Part print with two shaded views. Sizes in mm from the minimum x, y, z corner. Give positions to 0.01 mm unless a question says otherwise; leave off trailing zeros. Order: outer loops, then holes, each group sorted by start corner. A loop starts at its lowest first (then second) coordinate and runs counter-clockwise, first axis right, second up. Notation, with made-up numbers: M 15,81.25 L 43,81.25 A32 ccw 43,116.25 Z; hole C 83.5,-22.5 d4. An arc over 180 degrees is marked long. Return JSON: item names as keys, results as strings. Group by question number.
1. Slice it at B-B on z = 120. List the corners of the cut face in (x, y) (3 decimals).
2. Pin check, flat tips, straight feed: pin 1 (1 mm diameter, centred on x = 158.5, y = 2, fed in from -Z) (3 decimals); pin 2 (1 mm diameter, centred on y = 2, z = 59, fed in from +X) (3 decimals); pin 3 (0.7 mm diameter, centred on x = 2, y = 1, fed in from -Z). Stop position of each tip, or through.
3. Wall check: probe 1 along Z at (x, y) = (83, 2.3) (3 decimals); probe 2 along X at (y, z) = (0.7, 117.5) (3 decimals). Give the ranges that are in metal, low to high. Write a range as [from, to].
4. Slice it at A-A on x = 119. List the corners of the cut face in (y, z) (3 decimals).
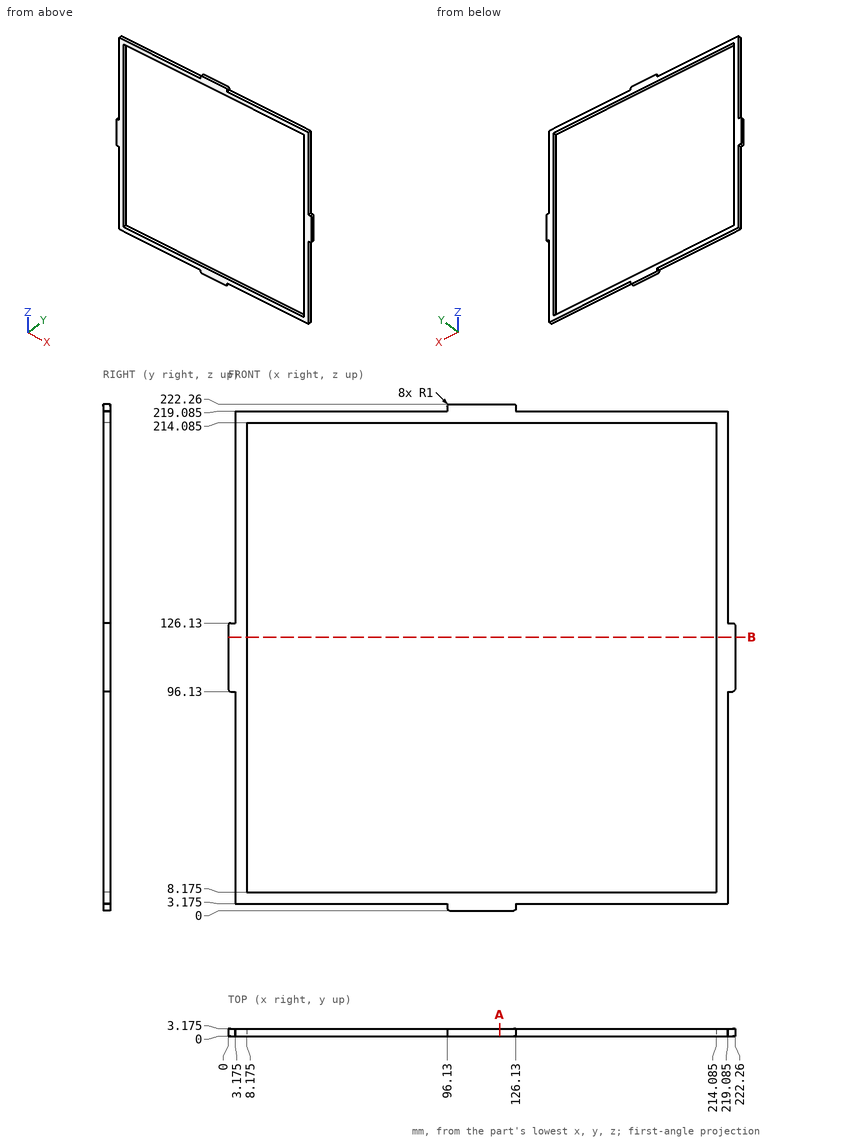
Result:
{
 "1": {"outline": "M 0,0 L 8.175,0 L 8.175,3.175 L 0,3.175 Z; M 214.085,0 L 222.26,0 L 222.26,3.175 L 214.085,3.175 Z"},
 "2": {"pin 1": "stops at z = 3.175", "pin 2": "stops at x = 219.085", "pin 3": "stops at z = 96.13"},
 "3": {"probe 1": "z = [3.175, 8.175], [214.085, 219.085]", "probe 2": "x = [0, 8.175], [214.085, 222.26]"},
 "4": {"outline": "M 0,0 L 3.175,0 L 3.175,8.175 L 0,8.175 Z; M 0,214.085 L 3.175,214.085 L 3.175,222.26 L 0,222.26 Z"}
}
